Could you check a few things on this model? Use its own coordinates, in mm. Give positions to 0.01 mm unless a question says otherwise; leave off trailing zeros. Order: outer loops, then holes, each group sorted by start corner. A loop starts at its lowest first (then second) coordinate and runs counter-clockwise, first axis right, second up.
(1) Will these pins go through, and if not, where does the flat tip stop? pin 1 (3 mm diameter, centred on x = -1.5, y = -6.5, fed in from +Z); pin 2 (1.9 mm diameter, centred on x = 0, z = -0.5, fed in from +Y).
(2) If I drill on probe 1 along Y at (x, z) = (0, -0.25); probe 2 along Y at (x, z) = (1.5, -2.5); probe 3 along X at (y, z) = (-1.75, -1), over which ranges is the centre line in solid material (lowest first)?
(3) Imagine slicing it at A-A, the plane y = -4. Write out the boundary of the cut face in (x, z), then the cut area to 3 significant figures.
(4) If we mould it in two halves opening along X, with no side actions, what happens to faces 1 (the flat face through (0, 1.2, 0)), 2 (the cylindrical face through (-0.575, -3.961, -1.386)), 3 (the flat face through (0, -10, 0))? For each: released by +X, released by -X, zero draft, split by the parting line, or undercut.
from build123d import *

# Parameters (mm, degrees)
SKETCH2_R           = 1.5
BOSS_EXTRUDE1_DEPTH = 10
CUT_EXTRUDE1_DEPTH  = 0.5
FILLET1_R           = 0.2
FILLET3_R           = 2


with BuildPart() as part:
    # Sketch1 → Revolve1 (revolve)
    with BuildSketch(Plane.XY, mode=Mode.PRIVATE) as revolve1_sk:
        Polygon((0, 0), (0, 1.7), (3.2, 1.7), (1.5, 0), align=None)
    revolve(revolve1_sk.sketch.rotate(Axis((0, 50, 0), (0, -1, 0)), 90), axis=Axis((0, 50, 0), (0, -1, 0)))

    # Sketch2 → Boss-Extrude1 (add)
    with BuildSketch(Plane.XZ):
        with Locations(Location((0, 0, 0), (0, 0, 270))):
            Circle(SKETCH2_R)
    extrude(amount=BOSS_EXTRUDE1_DEPTH)

    # Sketch3 → Cut-Revolve1 (revolve, cut)
    with BuildSketch(Plane.XY, mode=Mode.PRIVATE) as cut_revolve1_sk:
        Polygon((1.5, -8.2), (1.2, -10), (1.5, -10), align=None)
    revolve(cut_revolve1_sk.sketch.rotate(Axis((0, 0, 0), (0, -1, 0)), 180), axis=Axis((0, 0, 0), (0, -1, 0)), mode=Mode.SUBTRACT)

    # Sketch4 → Cut-Extrude1 (cut)
    with BuildSketch(Plane(origin=(0, 1.7, 0), x_dir=(1, 0, 0), z_dir=(0, 1, 0))):
        Polygon((0, 1.152050808), (0.330273688, 0.58), (1, 0.58), (0.665136844, 0), (1, -0.58), (0.330273688, -0.58), (0, -1.152050808), (-0.330273688, -0.58), (-1, -0.58), (-0.665136844, 0), (-1, 0.58), (-0.330273688, 0.58), align=None)
    extrude(amount=-CUT_EXTRUDE1_DEPTH, mode=Mode.SUBTRACT)

    # Fillet1
    fillet1_edges = [part.edges().sort_by_distance(p)[0] for p in [
        (-0.330273688, 1.45, -0.58),
        (0, 1.45, -1.152050808),
        (0.330273688, 1.45, -0.58),
        (1, 1.45, -0.58),
        (0.665136844, 1.45, 0),
        (1, 1.45, 0.58),
        (0.330273688, 1.45, 0.58),
        (0, 1.45, 1.152050808),
        (-0.330273688, 1.45, 0.58),
        (-1, 1.45, 0.58),
        (-0.665136844, 1.45, 0),
        (-1, 1.45, -0.58),
    ]]
    fillet(fillet1_edges, radius=FILLET1_R)

    # Fillet3
    fillet3_edges = [part.edges().sort_by_distance(p)[0] for p in [
        (-1.060660172, -8.2, -1.060660172),
    ]]
    fillet(fillet3_edges, radius=FILLET3_R)


solid = part.part
Answer block:
1. pin 1: stops at z = 1.5
1. pin 2: stops at y = 1.7
2. probe 1: y = -10 to 1.2
2. probe 2: y = 1.42 to 1.7
2. probe 3: x = -1.12 to 1.12
3. outline: circle Ø3 at (0, 0)
3. area: 7.07 mm2
4. face 1: undercut
4. face 2: split by the parting line
4. face 3: zero draft
